Here's how the part is built. I have some questions about the finished solid (model axes, mm). A direction names the side the tool comes from. Coordinates: 2 decimals unless noted, no trailing zeros. Write each loop counter-clockwise with the first axis right and the second up, starting at its lowest first coordinate (ties: lowest second). Pieces come first, ordered by that corner, then holes.
(1) Thinking about a two-plate mould opening in X: for faces 1 (the flat face through (13.96, 23.73, 0.25)), 2 (the flat face through (-13.574, 23.955, 0.246)), 3 (the flat face through (11.447, -6.839, 0.246)), 4 (the flat face through (-7, 0, 0.5)), which applies, released by +X, released by -X, zero draft, split by the parting line, or undercut?
(2) Please list where these lines run through material, in increasing order: probe 1 along X at (y, z) = (-3, 0.1); probe 2 along X at (y, z) = (10, 0.35); probe 3 along Y at (x, z) = (2, 0.15).
(3) Imagine slicing it at A-A, the plane z = 0.2. State how many separate pieces and enclosed holes the cut face has, plus the area to 3 significant figures.
(4) Which directions (+Z, -Z, +X, -X, +Y, -Y) give clear straight access to the entire face, cutting with the end or side of a thin tool? Please do faces 5 (the flat face through (6.45, 1.84, 0.25)), 6 (the flat face through (13.574, -23.955, 0.246)).
(5) Imagine slicing it at D-D, the plane x = -17. List the corners of the cut face in (y, z) for me.
(6) For pin 1 Ø12 at (x, y) = (15, -6.5) entering from -Z, with a flat end and sliding along its axis, tell me the tip position at first contact or that it passes through.
(7) Imagine slicing it at B-B, the plane y = 4.5. List the corners of the cut face in (x, z) for me.
(8) Imagine slicing it at C-C, the plane x = -9. List the corners of the cut face in (y, z) for me, plus the area to 3 significant figures.
```python
from build123d import *

# Parameters (mm, degrees)
BOSS_EXTRUDE1_DEPTH = 0.5


with BuildPart() as part:
    # Sketch1 → Boss-Extrude1 (new body)
    with BuildSketch(Plane.XY):
        Polygon((27.53269207, 15.896007178), (0, 31.792014357), (-27.53269207, 15.896007178), (-27.53269207, -15.896007178), (0, -31.792014357), (27.53269207, -15.896007178), align=None)
        Polygon((23.094010768, 13.333333333), (15.396007178, 13.333333333), (19.245008973, 6.666666667), align=None, mode=Mode.SUBTRACT)
        Polygon((4.426352064, -19), (18.667658704, 5.666666667), (14.24130664, 13.333333333), (7.024428275, 0.833333333), (12.028130608, 0.833333333), (11.065880159, -0.833333333), (6.062177826, -0.833333333), (0, -11.333333333), (-6.062177826, -0.833333333), (-11.065880159, -0.833333333), (-12.028130608, 0.833333333), (-7.024428275, 0.833333333), (-14.24130664, 13.333333333), (-18.667658704, 5.666666667), (-4.426352064, -19), align=None, mode=Mode.SUBTRACT)
        Polygon((0, -9.333333333), (13.086606102, 13.333333333), (-13.086606102, 13.333333333), align=None, mode=Mode.SUBTRACT)
        Polygon((-23.094010768, 13.333333333), (-19.245008973, 6.666666667), (-15.396007178, 13.333333333), align=None, mode=Mode.SUBTRACT)
    extrude(amount=BOSS_EXTRUDE1_DEPTH)


solid = part.part
```
Recorded:
1. face 1: released by +X
1. face 2: released by -X
1. face 3: undercut
1. face 4: zero draft
2. probe 1: x = -27.53 to -13.66, -4.81 to -3.66, 3.66 to 4.81, 13.66 to 27.53
2. probe 2: x = -27.53 to -21.17, -17.32 to -16.17, -12.32 to -11.16, 11.16 to 12.32, 16.17 to 17.32, 21.17 to 27.53
2. probe 3: y = -30.64 to -19, -7.87 to -5.87, 13.33 to 30.64
3. separate pieces: 1
3. enclosed holes: 4
3. area: 1,820 mm2
4. face 5: +Z, -Z
4. face 6: +Z, -Z, +X, -Y
5. outline: (-21.98, 0) - (2.78, 0) - (2.78, 0.5) - (-21.98, 0.5) - close; (8.56, 0) - (10.56, 0) - (10.56, 0.5) - (8.56, 0.5) - close; (13.33, 0) - (21.98, 0) - (21.98, 0.5) - (13.33, 0.5) - close
6. pin 1: stops at z = 0
7. outline: (-27.53, 0) - (-17.99, 0) - (-17.99, 0.5) - (-27.53, 0.5) - close; (-9.14, 0) - (-7.99, 0) - (-7.99, 0.5) - (-9.14, 0.5) - close; (7.99, 0) - (9.14, 0) - (9.14, 0.5) - (7.99, 0.5) - close; (17.99, 0) - (27.53, 0) - (27.53, 0.5) - (17.99, 0.5) - close
8. outline: (-26.6, 0) - (-11.08, 0) - (-11.08, 0.5) - (-26.6, 0.5) - close; (-0.83, 0) - (0.83, 0) - (0.83, 0.5) - (-0.83, 0.5) - close; (4.26, 0) - (6.26, 0) - (6.26, 0.5) - (4.26, 0.5) - close; (13.33, 0) - (26.6, 0) - (26.6, 0.5) - (13.33, 0.5) - close
8. area: 16.2 mm2
